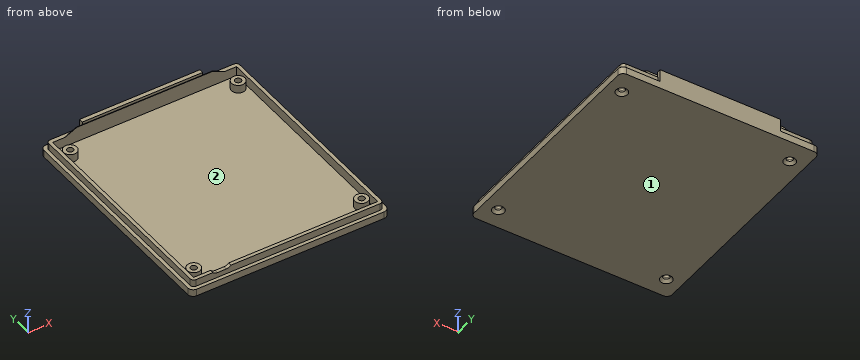
```python
from build123d import *

# Parameters (mm, degrees)
DODANIE_WYCI_GNI_CIE1_DEPTH      = 0.5
DODANIE_WYCI_GNI_CIE1_DEPTH_BACK = 2
DODANIE_WYCI_GNI_CIE2_DEPTH      = 5.5
DODANIE_WYCI_GNI_CIE3_DEPTH      = 1.5
ZAOKR_GLENIE1_R                  = 2
SZKIC6_W                         = 67.685530181
SZKIC6_H                         = 2.4
DODANIE_WYCI_GNI_CIE4_DEPTH      = 8.59
DODANIE_WYCI_GNI_CIE5_DEPTH      = 8.59
WYTNIJ_WYCI_GNI_CIE1_DEPTH       = 5.5
SZKIC13_R                        = 3.75
SZKIC13_R_2                      = 1.75
DODANIE_WYCI_GNI_CIE7_DEPTH      = 4.57
SZKIC13_3_R                      = 1.75
WYTNIJ_WYCI_GNI_CIE2_DEPTH       = 90.286037732
WYTNIJ_WYCI_GNI_CIE3_DEPTH       = 2
SFAZOWANIE1_SIZE                 = 1.5
ZAOKR_GLENIE2_R                  = 3


with BuildPart() as part:
    # Szkic3 → Dodanie-wyciągnięcie1 (new, two sides: drawn at the far end of the back side and taken through both)
    with BuildSketch(Plane(origin=(0, 0, -8.74), x_dir=(-1, 0, 0), z_dir=(0, 0, -1)).offset(-DODANIE_WYCI_GNI_CIE1_DEPTH_BACK)):
        Polygon((55.692889856, -69.15246634), (55.692892168, 60.038263946), (-55.811722529, 60.038263946), (-55.811687853, -69.161116694), align=None)
    extrude(amount=DODANIE_WYCI_GNI_CIE1_DEPTH + DODANIE_WYCI_GNI_CIE1_DEPTH_BACK)

    # Szkic4 → Dodanie-wyciągnięcie2 (add)
    with BuildSketch(Plane.XY.offset(-6.74)):
        Polygon((53.802147291, -67.151419689), (53.80218089, 58.038263946), (-53.683348754, 58.038263946), (-53.683348754, -67.143081129), align=None)
        Polygon((51.802147827, -65.151264526), (51.802180354, 56.038263946), (-51.683348754, 56.038263946), (-51.683348754, -65.14323628), align=None, mode=Mode.SUBTRACT)
    extrude(amount=DODANIE_WYCI_GNI_CIE2_DEPTH)

    # Szkic4<3> → Dodanie-wyciągnięcie3 (add)
    with BuildSketch(Plane.XY.offset(-6.74)):
        Polygon((-55.692892168, 60.038263946), (-55.692889856, -69.15246634), (55.811687853, -69.161116694), (55.811722529, 60.038263946), align=None)
        Polygon((-53.683348754, -67.143081129), (-53.683348754, 58.038263946), (53.80218089, 58.038263946), (53.802147291, -67.151419689), align=None, mode=Mode.SUBTRACT)
    extrude(amount=DODANIE_WYCI_GNI_CIE3_DEPTH)

    # Zaokrąglenie1
    zaokr_glenie1_edges = [part.edges().sort_by_distance(p)[0] for p in [
        (53.80218089, 58.038263946, -3.24),
        (-53.683348754, 58.038263946, -3.24),
        (-53.683348754, -67.143081129, -3.24),
        (53.802147291, -67.151419689, -3.24),
    ]]
    fillet(zaokr_glenie1_edges, radius=ZAOKR_GLENIE1_R)

    # Szkic6 → Dodanie-wyciągnięcie4 (add)
    with BuildSketch(Plane.XY.offset(-6.74)):
        with Locations((0.159416337, 58.838263946)):
            Rectangle(SZKIC6_W, SZKIC6_H)
    extrude(amount=DODANIE_WYCI_GNI_CIE4_DEPTH)

    # Szkic7 → Dodanie-wyciągnięcie5 (add)
    with BuildSketch(Plane.XY.offset(-6.74)):
        Polygon((-51.683348754, 55.738263946), (51.802180273, 55.738263946), (51.802180354, 56.038263946), (-51.683348754, 56.038263946), align=None)
    extrude(amount=DODANIE_WYCI_GNI_CIE5_DEPTH)

    # Szkic9 → Wytnij-wyciągnięcie1 (cut)
    with BuildSketch(Plane.XZ.offset(-55.738263946)):
        Polygon((51.802180273, 1.85), (38.175466286, 1.85), (44.80199267, -1.24), (51.80199267, -1.24), (51.802180273, -1.24), align=None)
        Polygon((-38.056977527, 1.85), (-51.683348754, 1.85), (-51.683348754, -1.24), (-44.683503911, -1.24), align=None)
    extrude(amount=-WYTNIJ_WYCI_GNI_CIE1_DEPTH, mode=Mode.SUBTRACT)

    # Szkic13 → Dodanie-wyciągnięcie7 (add)
    # profile 1 of 4: a face of its own
    with BuildSketch(Plane.XY.offset(-6.74)):
        with Locations((-47.14, 47.6022)):
            Circle(SZKIC13_R)
        with Locations((-47.14, 47.6022)):
            Circle(SZKIC13_R_2, mode=Mode.SUBTRACT)
    # profile 2 of 4: a face of its own
    with BuildSketch(Plane.XY.offset(-6.74)):
        with Locations((47.352, 47.6022)):
            Circle(SZKIC13_R)
        with Locations((47.352, 47.6022)):
            Circle(SZKIC13_R_2, mode=Mode.SUBTRACT)
    # profile 3 of 4: a face of its own
    with BuildSketch(Plane.XY.offset(-6.74)):
        with Locations((-47.14, -58.1478)):
            Circle(SZKIC13_R)
        with Locations((-47.14, -58.1478)):
            Circle(SZKIC13_R_2, mode=Mode.SUBTRACT)
    # profile 4 of 4: a face of its own
    with BuildSketch(Plane.XY.offset(-6.74)):
        with Locations((47.352, -58.1478)):
            Circle(SZKIC13_R)
        with Locations((47.352, -58.1478)):
            Circle(SZKIC13_R_2, mode=Mode.SUBTRACT)
    extrude(amount=DODANIE_WYCI_GNI_CIE7_DEPTH)

    # Szkic13<3> → Wytnij-wyciągnięcie2 (cut, through all)
    with BuildSketch(Plane.XY.offset(-6.74)):
        with Locations((-47.14, -58.1478)):
            Circle(SZKIC13_3_R)
        with Locations((-47.14, 47.6022)):
            Circle(SZKIC13_3_R)
        with Locations((47.352, 47.6022)):
            Circle(SZKIC13_3_R)
        with Locations((47.352, -58.1478)):
            Circle(SZKIC13_3_R)
    extrude(amount=-WYTNIJ_WYCI_GNI_CIE2_DEPTH, mode=Mode.SUBTRACT)

    # Szkic18 → Wytnij-wyciągnięcie3 (cut)
    with BuildSketch(Plane(origin=(-0.00520918, -67.147245397, 0), x_dir=(0.999999996990791, -7.757846392237927e-05, 0), z_dir=(-7.757846392237927e-05, -0.999999996990791, 0))):
        with BuildLine():
            ThreePointArc((-42.245261471, -1.24), (-41.074504923, -2.078778872), (-39.665102055, -2.375097025))
            Line((-39.665102055, -2.375097025), (-34.665098037, -2.375097025))
            ThreePointArc((-34.665098037, -2.375097025), (-33.255694971, -2.078778946), (-32.084938256, -1.24))
            Line((-32.084938256, -1.24), (-42.245261471, -1.24))
        make_face()
    extrude(amount=-WYTNIJ_WYCI_GNI_CIE3_DEPTH, mode=Mode.SUBTRACT)

    # Sfazowanie1
    sfazowanie1_edges = [part.edges().sort_by_distance(p)[0] for p in [
        (45.602, -58.1478, -9.24),
        (45.602, 47.6022, -9.24),
        (-48.89, 47.6022, -9.24),
        (-48.89, -58.1478, -9.24),
    ]]
    chamfer(sfazowanie1_edges, length=SFAZOWANIE1_SIZE)

    # Zaokrąglenie2
    zaokr_glenie2_edges = [part.edges().sort_by_distance(p)[0] for p in [
        (55.811687853, -69.161116694, -7.24),
        (55.811722529, 60.038263946, -7.24),
        (-55.692892168, 60.038263946, -7.24),
        (-55.692889856, -69.15246634, -7.24),
    ]]
    fillet(zaokr_glenie2_edges, radius=ZAOKR_GLENIE2_R)


solid = part.part
```
Check sheet for the modelled part. Datum: model origin and axes. Units: mm. Face numbers are marked on the shaded views. Coordinates: 2 decimals unless noted, no trailing zeros. Loops run counter-clockwise (first coordinate to the right, second up) from the corner with the lowest first, then second, coordinate; pieces in that order, holes last. Notation, with made-up numbers: M 16.5,68.25 L 24.5,68.25 A19 ccw 24.5,98.25 Z; hole C 71.5,-3.75 d8. An arc over 180 degrees is marked long. Answer as a JSON object with one key per item and string values.
1. Sectioned sample at D-D on x = -19. Record the cut outline in (y, z), and give its area (3 significant figures).
Outcome:
{"outline": "M -69.16,-9.24 L 60.04,-9.24 L 60.04,1.85 L 57.64,1.85 L 57.64,-1.24 L 56.04,-1.24 L 56.04,1.85 L 55.74,1.85 L 55.74,-6.74 L -65.15,-6.74 L -65.15,-1.24 L -67.15,-1.24 L -67.15,-5.24 L -69.16,-5.24 Z", "area": "369 mm²"}
2. Scan lines: L1, parallel to Y at x = -23, z = -1.5; L2, parallel to X at y = -25.5, z = -2.5; L3, parallel to Y at x = -11.5, z = -5.5. Record each from-to range of solid material in increasing order. Write a range as from..to.
Outcome:
{"L1": "-67.15..-65.15, 55.74..60.04", "L2": "-53.68..-51.68, 51.8..53.8", "L3": "-69.16..-65.15, 55.74..60.04"}
3. Sectioned sample at C-C on x = 42. Record the cut outline in (y, z), and give its area (3 significant figures).
Outcome:
{"outline": "M -69.16,-9.24 L 60.04,-9.24 L 60.04,-5.24 L 58.04,-5.24 L 58.04,-1.24 L 56.04,-1.24 L 56.04,0.07 L 55.74,0.07 L 55.74,-6.74 L -65.15,-6.74 L -65.15,-1.24 L -67.15,-1.24 L -67.15,-5.24 L -69.16,-5.24 Z", "area": "353 mm²"}
4. Sectioned sample at B-B on x = -47.14. Count the separate pieces of the cut face and the enclosed holes in it, and give its area (3 significant figures).
Outcome:
{"separate pieces": "3", "enclosed holes": "0", "area": "367 mm²"}
5. Depth check by flat-ended pin: P1, Ø5, axis at x = 28, z = -1.5, coming from the -Y side; P2, Ø1.9, axis at y = 59.5, z = -1, coming from the +X side; P3, Ø3, axis at y = -17.5, z = -3, coming from the +X side. Enter the tip coordinate at first touch or a pass-through.
Outcome:
{"P1": "y = -67.15", "P2": "x = 34", "P3": "x = 53.8"}
6. Sectioned sample at A-A on y = 22.5. Record the cut outline in (x, z), and give its area (3 significant figures).
Outcome:
{"outline": "M -55.69,-9.24 L 55.81,-9.24 L 55.81,-5.24 L 53.8,-5.24 L 53.8,-1.24 L 51.8,-1.24 L 51.8,-6.74 L -51.68,-6.74 L -51.68,-1.24 L -53.68,-1.24 L -53.68,-5.24 L -55.69,-5.24 Z", "area": "307 mm²"}
7. Release check for a two-part mould opening along X. For the marked faces 1 and 2 record: pulls with the +X half, pulls with the -X half, needs draft (parallel to the pull), parting line crosses it, or undercut.
Outcome:
{"face 1": "needs draft", "face 2": "undercut"}
